from build123d import *

# Parameters (mm, degrees)
F0_W     = 3.81
F0_H     = 3.81
F0_H_2   = 30.2708674201
F0_H_3   = 4.0191325799
F1_DEPTH = 17.78
F2_W     = 152.4
F2_H     = 38.1
F3_DEPTH = 2.54


with BuildPart() as f1:
    # F0 (on Top) → F1 (new body)
    with BuildSketch(Plane.XY):
        Polygon((-72.39, 15.24), (72.39, 15.24), (72.39, 19.05), (-68.58, 19.05), (-72.39, 19.05), align=None)
        with Locations((-74.295, 17.145)):
            Rectangle(F0_W, F0_H)
        with Locations((-74.295, 0.1045662899)):
            Rectangle(F0_W, F0_H_2)
        with Locations((-74.295, -17.0404337101)):
            Rectangle(F0_W, F0_H_3)
        Polygon((-71.3768037915, -19.05), (72.39, -19.05), (72.39, -15.0308674201), (-72.39, -15.0308674201), (-72.39, -19.05), align=None)
        with Locations((74.295, 0.1045662899)):
            Rectangle(F0_W, F0_H_2)
        Polygon((72.39, -19.05), (76.2, -19.05), (76.2, -18.8408674201), (76.2, -15.0308674201), (72.39, -15.0308674201), align=None)
        with Locations((74.295, 17.145)):
            Rectangle(F0_W, F0_H)
    extrude(amount=F1_DEPTH)

    # F2 (on Top) → F3 (join)
    with BuildSketch(Plane.XY):
        Rectangle(F2_W, F2_H)
    extrude(amount=F3_DEPTH)


solid = f1.part
Geometry: final body of the model. Coordinates: model frame, mm. A direction names the side the tool comes from. Give positions to 0.01 mm unless a question says otherwise; leave off trailing zeros. Write each loop counter-clockwise with the first axis right and the second up, starting at its lowest first coordinate (ties: lowest second). Pieces come first, ordered by that corner, then holes. Notation, with made-up numbers: (-12.5, 27.25) -> (40.5, 27.25) arc R4 cw to (40.5, 33.25) -> close; hole circle Ø1 at (74, 44). An arc over 180 degrees is marked (long way). Answer as a JSON object with one key per item and string values.
1. Cut plane A-A on x = 37. Output: boundary loops of the cut face in (y, z), and give its area (3 significant figures).
Ans:
{"outline": "(-19.05, 0) -> (19.05, 0) -> (19.05, 17.78) -> (15.24, 17.78) -> (15.24, 2.54) -> (-15.03, 2.54) -> (-15.03, 17.78) -> (-19.05, 17.78) -> close", "area": "216 mm^2"}
2. Cut plane C-C on y = 8.5. Output: boundary loops of the cut face in (x, z).
Ans:
{"outline": "(-76.2, 0) -> (76.2, 0) -> (76.2, 17.78) -> (72.39, 17.78) -> (72.39, 2.54) -> (-72.39, 2.54) -> (-72.39, 17.78) -> (-76.2, 17.78) -> close"}
3. Ray query, probe 1 along Y at (x, z) = (-46, 8.25); probe 2 along X at (y, z) = (-8.5, 11.25); probe 3 along Z at (x, y) = (-22, -3.5). Return the intervals inside material, ascending. Write a range as from..to.
Ans:
{"probe 1": "y = -19.05..-15.03, 15.24..19.05", "probe 2": "x = -76.2..-72.39, 72.39..76.2", "probe 3": "z = 0..2.54"}
4. Access query for faces 4 (the flat face through (-1, 0, 0)), 5 (the flat face through (-72.39, 0, 10)). Directions: +Z, -Z, +X, -X, +Y, -Y. A direction counts if a zero-diameter tool reaches every point of the face in a straight line with its end or side. Return the directions, or none.
Ans:
{"face 4": "-Z, +X, -X, +Y, -Y", "face 5": "+Z"}
5. Mould query, pull axis X, two halves, no side actions, for faces 1 (the flat face through (76.2, 0, 9)), 2 (the flat face through (-1, -19.05, 9)), 3 (the flat face through (1, -15.031, 10)). Classes: pulls with the +X half, pulls with the -X half, needs draft (parallel to the pull), parting line crosses it, or undercut.
Ans:
{"face 1": "pulls with the +X half", "face 2": "needs draft", "face 3": "undercut"}
6. Contact query for a flat-ended pin moving along its axis: pin 1 (4 mm diameter, centred on x = 46.5, y = -10.5, fed in from +Z). Output: stop coordinate, or through.
Ans:
{"pin 1": "stops at z = 2.54"}
7. Cut plane B-B on z = 6. Output: boundary loops of the cut face in (x, y).
Ans:
{"outline": "(-76.2, -19.05) -> (76.2, -19.05) -> (76.2, 19.05) -> (-76.2, 19.05) -> close; hole (-72.39, -15.03) -> (72.39, -15.03) -> (72.39, 15.24) -> (-72.39, 15.24) -> close"}
